```python
from build123d import *

# Parameters (mm, degrees)
SKETCH003_R      = 3
EXTRUDE004_DEPTH = 15.5
EXTRUDE002_DEPTH = 2
SKETCH001_W      = 40
SKETCH001_H      = 19.95
EXTRUDE001_DEPTH = 35


with BuildPart() as extrude004:
    # Sketch003 → Extrude004 (new body)
    with BuildSketch(Plane.XY):
        Circle(SKETCH003_R)
    extrude(amount=EXTRUDE004_DEPTH)


with BuildPart() as fusion:
    # Sketch → Extrude002 (new body)
    with BuildSketch(Plane.XY):
        with BuildLine():
            Line((-37.8, 9.975), (17.8, 9.975))
            Line((17.8, 9.975), (17.8, 6.8))
            Line((15.587451, 6.8), (17.8, 6.8))
            ThreePointArc((15.587451, 6.8), (11.6, 5), (15.587451, 3.2))
            Line((15.587451, 3.2), (17.8, 3.2))
            Line((17.8, -3.2), (17.8, 3.2))
            Line((15.587451, -3.2), (17.8, -3.2))
            ThreePointArc((15.587451, -3.2), (11.6, -5), (15.587451, -6.8))
            Line((15.587451, -6.8), (17.8, -6.8))
            Line((17.8, -6.8), (17.8, -9.975))
            Line((17.8, -9.975), (-37.8, -9.975))
            Line((-37.8, -9.975), (-37.8, -6.8))
            Line((-37.8, -6.8), (-35.587451, -6.8))
            ThreePointArc((-35.587451, -6.8), (-31.6, -5), (-35.587451, -3.2))
            Line((-37.8, -3.2), (-35.587451, -3.2))
            Line((-37.8, 3.2), (-37.8, -3.2))
            Line((-35.587451, 3.2), (-37.8, 3.2))
            ThreePointArc((-35.587451, 3.2), (-31.6, 5), (-35.587451, 6.8))
            Line((-37.8, 6.8), (-35.587451, 6.8))
            Line((-37.8, 9.975), (-37.8, 6.8))
        make_face()
    extrude(amount=EXTRUDE002_DEPTH)

    # Fusion: union Extrude004
    add(extrude004.part)


with BuildPart() as fusion001:
    # Sketch001 → Extrude001 (new body)
    with BuildSketch(Plane.XY.offset(9.3)):
        with Locations((-10, 0)):
            Rectangle(SKETCH001_W, SKETCH001_H)
    extrude(amount=-EXTRUDE001_DEPTH)

    # Fusion001: union Fusion
    add(fusion.part)


solid = fusion001.part
```
Can you work these out from the model? Positions are in its coordinate system, mm. A direction names the side the tool comes from. Give positions to 0.01 mm unless a question says otherwise; leave off trailing zeros. Order: outer loops, then holes, each group sorted by start corner. A loop starts at its lowest first (then second) coordinate and runs counter-clockwise, first axis right, second up. Notation, with made-up numbers: (-27, -11) - (-1, -11) arc R19 cw to (-1, 0) - close; hole circle Ø10 at (76, -14). An arc over 180 degrees is marked (long way). Use a Markdown table: item, result. Add a question column.
Q1. On a 3-axis mill with a long thin cutter (end or side, diameter ignored), from which of +Z, -Z, +X, -X, +Y, -Y can I reach the whole of each face in a straight line? I mean faces 1 (the flat face through (-33, 0, 2)), 2 (the flat face through (-37, 6.8, 1)), 3 (the cylindrical face through (-3, 0, 12)). Say none if no direction works.
Q2. If we section it at D-D on z = 10: Write out the boundary of the cut face in (x, y), plus the area to 3 significant figures.
Q3. If we mould it in two halves opening along X, with no side actions, what happens to faces 4 (the flat face through (-37.8, -8, 1)), 5 (the flat face through (-37, 3.2, 1)), 6 (the cylindrical face through (11.6, 5.08, 0.99)), 7 (the cylindrical face through (11.6, -4.92, 0.99))? For each: released by +X, released by -X, zero draft, split by the parting line, or undercut.
Q4. If we section it at A-A on x = -34: Write out the boundary of the cut face in (y, z) (3 decimals), plus the area to 3 significant figures.
Q5. If we section it at C-C on y = -8.5: Write out the boundary of the cut face in (x, z).
Q6. If we section it at B-B on x = 0: Write out the boundary of the cut face in (y, z) (3 decimals).
Q7. I'm going to push flat-ended pins straight in: pin 1 (1 mm diameter, centred on y = -6, z = -6, fed in from +X); pin 2 (8 mm diameter, centred on y = -0.5, z = 6.5, fed in from -X); pin 3 (2 mm diameter, centred on x = 11.5, y = -2, fed in from +Z). Where does each tip first touch, or does it pass through?
Q8. Please list where these lines run through material, in increasing order: line 1 along Y through (x, z) = (14, 1) (3 decimals); line 2 along X through (y, z) = (-7.5, -11.5); line 3 along Z through (x, y) = (-33, 0.5).
Answers follow:
| question | item | result |
|---|---|---|
| 1 | face 1 | +Z, -X, +Y, -Y |
| 1 | face 2 | +Z, -Z, -X |
| 1 | face 3 | +Z |
| 2 | outline | circle Ø6 at (0, 0) |
| 2 | area | 28.3 mm^2 |
| 3 | face 4 | released by -X |
| 3 | face 5 | zero draft |
| 3 | face 6 | undercut |
| 3 | face 7 | undercut |
| 4 | outline | (-9.975, 0) - (-7.4, 0) - (-7.4, 2) - (-9.975, 2) - close; (-2.6, 0) - (2.6, 0) - (2.6, 2) - (-2.6, 2) - close; (7.4, 0) - (9.975, 0) - (9.975, 2) - (7.4, 2) - close |
| 4 | area | 20.7 mm^2 |
| 5 | outline | (-37.8, 0) - (-30, 0) - (-30, -25.7) - (10, -25.7) - (10, 0) - (17.8, 0) - (17.8, 2) - (10, 2) - (10, 9.3) - (-30, 9.3) - (-30, 2) - (-37.8, 2) - close |
| 6 | outline | (-9.975, -25.7) - (9.975, -25.7) - (9.975, 9.3) - (3, 9.3) - (3, 15.5) - (-3, 15.5) - (-3, 9.3) - (-9.975, 9.3) - close |
| 7 | pin 1 | stops at x = 10 |
| 7 | pin 2 | stops at x = -30 |
| 7 | pin 3 | stops at z = 2 |
| 8 | line 1 | y = -9.975 to -7.4, -2.6 to 2.6, 7.4 to 9.975 |
| 8 | line 2 | x = -30 to 10 |
| 8 | line 3 | z = 0 to 2 |
